from build123d import *

# Parameters (mm, degrees)
F1_DEPTH = 25.4
F2_R     = 3.175
F3_R     = 3.175


with BuildPart() as f1:
    # F0 (on Front) → F1 (new body)
    with BuildSketch(Plane.XZ):
        with BuildLine():
            ThreePointArc((0, 152.4), (-107.763073, -107.763073), (152.4, 0))
            ThreePointArc((152.4, 0), (126.804465, 84.53631), (58.615385, 140.676923))
            ThreePointArc((58.615385, 140.676923), (29.888099, 149.440495), (0, 152.4))
        make_face()
        with BuildLine():
            ThreePointArc((0, 152.4), (29.888099, 149.440495), (58.615385, 140.676923))
            Line((58.615385, 140.676923), (0, 165.1))
            Line((0, 165.1), (0, 152.4))
        make_face()
    extrude(amount=F1_DEPTH)

    # F2
    f2_edges = [f1.edges().sort_by_distance(p)[0] for p in [
        (0, -12.7, 152.4),
    ]]
    fillet(f2_edges, radius=F2_R)

    # F3
    f3_edges = [f1.edges().sort_by_distance(p)[0] for p in [
        (0, -12.7, 165.1),
    ]]
    fillet(f3_edges, radius=F3_R)


solid = f1.part
Read the model definition and answer for the solid it produces. Units are mm, in the model's axes. Round coordinates to 2 decimals unless told otherwise and drop trailing zeros. Write each loop counter-clockwise with the first axis right and the second up, starting at its lowest first coordinate (ties: lowest second). Pieces come first, ordered by that corner, then holes.
1. Determine the mould class of faces 1 (the face through (-2, -25.4, 8)), 2 (the face through (31.885, -12.522, 151.814)), 3 (the face through (-2, 0, 8)) for opening direction Y: pulls with the +Y half, pulls with the -Y half, needs draft (parallel to the pull), parting line crosses it, or undercut.
2. The part is cut by section C-C, the plane x = -75. Determine the outline of the cut face in (y, z), then the cut area to 3 significant figures.
3. Given pin 1 Ø3 at (x, y) = (57, -14.5) entering from -Z; pin 2 Ø1 at (x, y) = (-16.5, -20.5) entering from +Z; pin 3 Ø5.5 at (y, z) = (-6.5, 157) entering from -X, each flat-ended and moving along its own axis, determine where each tip first touches the part or whether it passes through.
4. Straight lines are drawn through the part: L1, parallel to Z at x = -21, y = -12.5; L2, parallel to Z at x = -102.5, y = -9.75; L3, parallel to X at y = -8.75, z = -8.5. For each, find the intervals that lie inside material, in ascending order.
5. The part is cut by section B-B, the plane z = -81. Determine the outline of the cut face in (x, y).
Values:
1. face 1: pulls with the -Y half
1. face 2: needs draft
1. face 3: pulls with the +Y half
2. outline: (-25.4, -132.67) - (0, -132.67) - (0, 132.67) - (-25.4, 132.67) - close
2. area: 6,740 mm2
3. pin 1: stops at z = -141.93
3. pin 2: stops at z = 151.56
3. pin 3: stops at x = -0.28
4. L1: z = -150.95 to 150.95
4. L2: z = -112.78 to 112.78
4. L3: x = -152.16 to 152.16
5. outline: (-129.09, -25.4) - (129.09, -25.4) - (129.09, 0) - (-129.09, 0) - close
